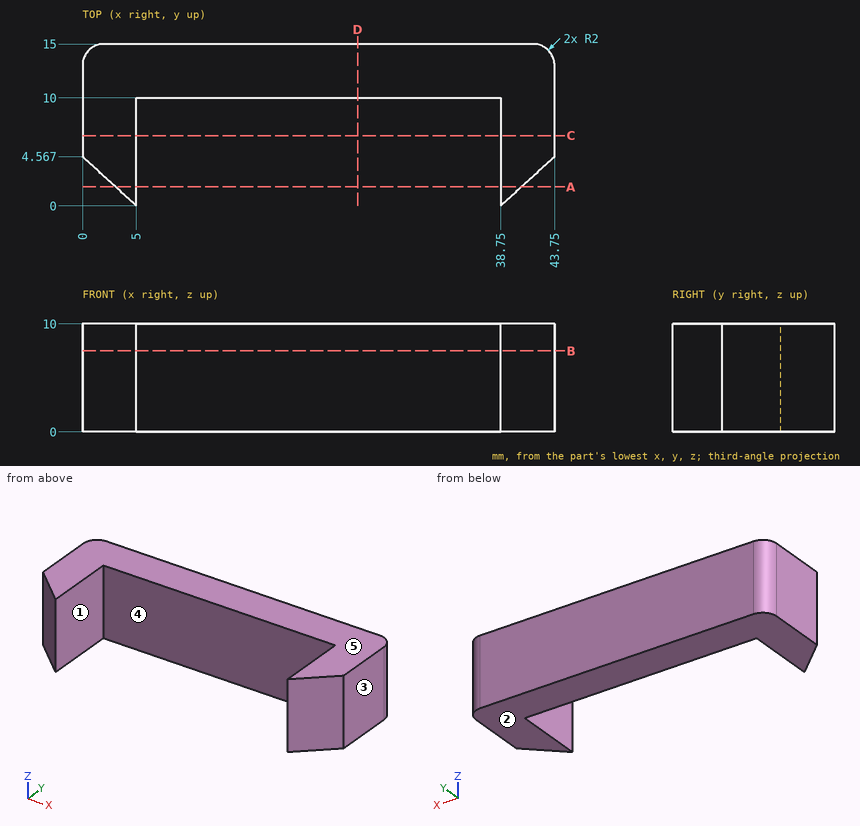
Input: dimensioned drawing with shaded views. Units: mm. Origin: part minimum x, y, z. A direction names the side the tool comes from. Give positions to 0.01 mm unless a question says otherwise; leave off trailing zeros. Loops run counter-clockwise (first coordinate to the right, second up) from the corner with the lowest first, then second, coordinate; pieces in that order, holes last. Notation, with made-up numbers: (67.25, -29.5) -> (120.25, -29.5) arc R18 ccw to (120.25, -25.5) -> close; hole circle Ø11 at (1.5, -26.75). An arc over 180 degrees is marked (long way). Use a Markdown table: item, result.
Q1. Section query C-C, the plane y = 6.5. Return the cut outline in (x, z).
Entries:
| item | result |
|---|---|
| outline | (0, 0) -> (5, 0) -> (5, 10) -> (0, 10) -> close; (38.75, 0) -> (43.75, 0) -> (43.75, 10) -> (38.75, 10) -> close |
Q2. Section query B-B, the plane z = 7.5. Return the cut outline in (x, y), plus the area to 3 significant figures.
Entries:
| item | result |
|---|---|
| outline | (0, 4.57) -> (5, 0) -> (5, 10) -> (38.75, 10) -> (38.75, 0) -> (43.75, 4.57) -> (43.75, 13) arc R2 ccw to (41.75, 15) -> (2, 15) arc R2 ccw to (0, 13) -> close |
| area | 294 mm² |
Q3. Ray query, probe 1 along X at (y, z) = (8.25, 3.5); probe 2 along Y at (x, z) = (37.5, 6.75); probe 3 along X at (y, z) = (3.25, 3.75). Return the intervals inside material, ascending. Write a range as from..to.
Entries:
| item | result |
|---|---|
| probe 1 | x = 0..5, 38.75..43.75 |
| probe 2 | y = 10..15 |
| probe 3 | x = 1.44..5, 38.75..42.31 |
Q4. First-contact query: P1, Ø1, axis at x = 9.5, z = 9, coming from the -Y side; P2, Ø1, axis at y = 4, z = 8.5, coming from the -X side; P3, Ø1, axis at y = 2, z = 7.5, coming from the +X side. Flat tips, straight axial feed; report the tip coordinate or a pass-through.
Entries:
| item | result |
|---|---|
| P1 | stops at y = 10 |
| P2 | stops at x = 0.07 |
| P3 | stops at x = 41.49 |
Q5. Section query A-A, the plane y = 1.75. Return the cut outline in (x, z).
Entries:
| item | result |
|---|---|
| outline | (3.08, 0) -> (5, 0) -> (5, 10) -> (3.08, 10) -> close; (38.75, 0) -> (40.67, 0) -> (40.67, 10) -> (38.75, 10) -> close |
Q6. Pull-direction query (X, two-part tool) for the marked faces 3, 4 and 5; classes: pulls with the +X half, pulls with the -X half, needs draft (parallel to the pull), parting line crosses it, or undercut.
Entries:
| item | result |
|---|---|
| face 3 | pulls with the +X half |
| face 4 | undercut |
| face 5 | needs draft |
Q7. Section query D-D, the plane x = 25.5. Return the cut outline in (y, z).
Entries:
| item | result |
|---|---|
| outline | (10, 0) -> (15, 0) -> (15, 10) -> (10, 10) -> close |
Q8. Access query for the marked faces 1 and 2. Directions: +Z, -Z, +X, -X, +Y, -Y. A direction counts if a zero-diameter tool reaches every point of the face in a straight line with its end or side. Return the directions, or none.
Entries:
| item | result |
|---|---|
| face 1 | +Z, -Z, -Y |
| face 2 | -Z, +X, -X, +Y, -Y |
